from build123d import *

# Parameters (mm, degrees)
SKETCH1_R           = 4.6
BOSS_EXTRUDE1_DEPTH = 5.35
BOSS_EXTRUDE2_START = 3
SKETCH1_3_R         = 2.2
BOSS_EXTRUDE2_DEPTH = 3
CHAMFER1_SIZE       = 0.75
CHAMFER2_SIZE       = 0.25


with BuildPart() as part:
    # Sketch1 → Boss-Extrude1 (new body)
    with BuildSketch(Plane(origin=(0, 0, 0), x_dir=(1, 0, 0), z_dir=(0, 1, 0))):
        with BuildLine():
            Line((0, 9), (22, 9))
            ThreePointArc((22, 9), (31, 0), (22, -9))
            Line((22, -9), (0, -9))
            ThreePointArc((0, -9), (-9, 0), (0, 9))
        make_face()
        with Locations(Location((0, 0, 0), (0, 0, 270))):
            Circle(SKETCH1_R, mode=Mode.SUBTRACT)
        with Locations(Location((22, 0, 0), (0, 0, 270))):
            Circle(SKETCH1_R, mode=Mode.SUBTRACT)
    extrude(amount=-BOSS_EXTRUDE1_DEPTH)

    # Sketch1_3 → Boss-Extrude2 (add)
    with BuildSketch(Plane(origin=(0, 0, 0), x_dir=(1, 0, 0), z_dir=(0, 1, 0)).offset(BOSS_EXTRUDE2_START)):
        with BuildLine():
            Line((22, 9), (0, 9))
            ThreePointArc((0, 9), (-9, 0), (0, -9))
            Line((0, -9), (22, -9))
            ThreePointArc((22, -9), (31, 0), (22, 9))
        make_face()
        with Locations(Location((0, 0, 0), (0, 0, 270))):
            Circle(SKETCH1_3_R, mode=Mode.SUBTRACT)
        with Locations(Location((22, 0, 0), (0, 0, 270))):
            Circle(SKETCH1_3_R, mode=Mode.SUBTRACT)
    extrude(amount=-BOSS_EXTRUDE2_DEPTH)

    # Chamfer1
    chamfer1_edges = [part.edges().sort_by_distance(p)[0] for p in [
        (0, -5.35, -4.6),
        (11, -5.35, 9),
        (11, 3, -9),
        (31, -5.35, 0),
        (11, 3, 9),
        (31, 3, 0),
        (-9, 3, 0),
        (11, -5.35, -9),
        (-9, -5.35, 0),
        (22, -5.35, -4.6),
    ]]
    chamfer(chamfer1_edges, length=CHAMFER1_SIZE)

    # Chamfer2
    chamfer2_edges = [part.edges().sort_by_distance(p)[0] for p in [
        (22, 3, -2.2),
        (0, 3, -2.2),
    ]]
    chamfer(chamfer2_edges, length=CHAMFER2_SIZE)


solid = part.part
The model under review builds one solid part; all positions refer to its coordinate system, in mm. A direction names the side the tool comes from. Give positions to 0.01 mm unless a question says otherwise; leave off trailing zeros. Write each loop counter-clockwise with the first axis right and the second up, starting at its lowest first coordinate (ties: lowest second). Pieces come first, ordered by that corner, then holes. Notation, with made-up numbers: M 14.25,1.5 L 19.25,1.5 A11 cw 19.25,20.5 Z; hole C -16.75,-4.75 d6. An arc over 180 degrees is marked long. One line per question, with ' | ' between items. Start each with the question number.
Item 1: We need section B-B on y = 1.5. Write out the cut boundary in (x, z).
Item 2: For faces 1 (the flat face through (-2.1, 0, -1.1)), 2 (the conical face through (30.37, 2.88, 0.18)), list the 3-axis set-ups (+Z, -Z, +X, -X, +Y, -Y) from which the entire face can be reached by the end or side of a thin tool; tool diameter is ignored.
Item 3: We need section A-A on z = 0. Give the number of separate pieces and of enclosed holes in the cut face, plus the area to 3 significant figures.
Item 4: We need section C-C on y = -2.5. Write out the cut boundary in (x, z), plus the area to 3 significant figures.
Item 5: Wall thickness on line 1 (X direction, y = -0.25, z = 0); line 2 (X direction, y = 1.3, z = 0); line 3 (Y direction, x = 26, z = -0.25): over which ranges is each line inside the solid? List them lowest first. Write a range as from..to.
Item 6: Draft analysis for pull direction Z (two halves, no side actions). For faces 3 (the conical face through (0, -5, -5)), 4 (the conical face through (22, -5, -5)), 5 (the flat face through (11, 3, 0)), 6 (the cylindrical face through (31, -1, 0)), state which applies: released by +Z, released by -Z, zero draft, split by the parting line, or undercut.
Item 7: For pin 1 (2.5 mm diameter, centred on x = 0, z = 0, fed in from +Y); pin 2 (2 mm diameter, centred on y = 2, z = 2.5, fed in from -X); pin 3 (1.5 mm diameter, centred on y = -4, z = -5.5, fed in from +X); pin 4 (3 mm diameter, centred on x = 1, z = 1, fed in from -Y), all flat-tipped, find the tip position at first contact; note any pin that passes through.
Results found:
1) outline: M 0,-9 L 22,-9 A9 ccw 22,9 L 0,9 A9 ccw Z; hole C 0,0 d4.4; hole C 22,0 d4.4
2) face 1: -Y | face 2: +X, +Y
3) separate pieces: 3 | enclosed holes: 0 | area: 207 mm2
4) outline: M 0,-9 L 22,-9 A9 ccw 22,9 L 0,9 A9 ccw Z; hole C 0,0 d9.2; hole C 22,0 d9.2 | area: 518 mm2
5) line 1: x = -9..-4.6, 4.6..17.4, 26.6..31 | line 2: x = -9..-2.2, 2.2..19.8, 24.2..31 | line 3: y = 0..3
6) face 3: undercut | face 4: undercut | face 5: zero draft | face 6: split by the parting line
7) pin 1: passes through | pin 2: stops at x = -8.87 | pin 3: stops at x = 29.64 | pin 4: stops at y = 0
